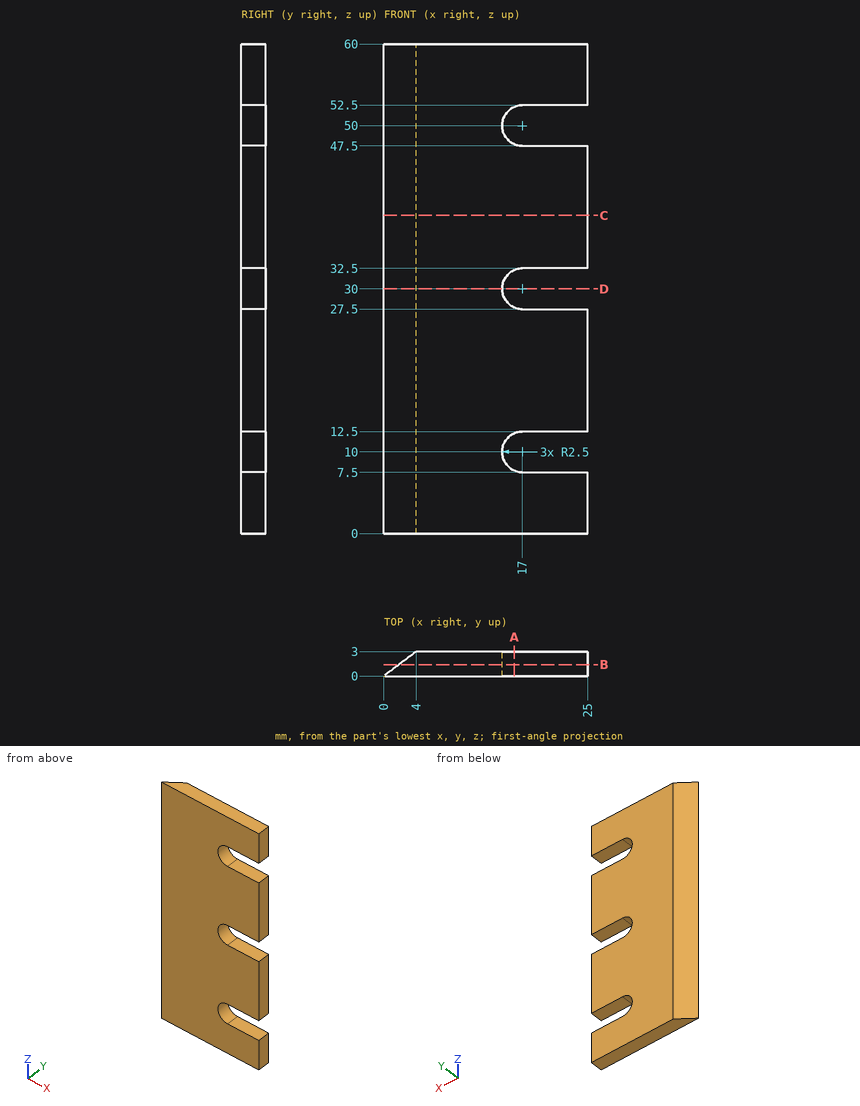
Could you check a few things on this drawing? It's one solid part, dimensions in mm from its lowest x, y, z. Give positions to 0.01 mm unless a question says otherwise; leave off trailing zeros. Write each loop counter-clockwise with the first axis right and the second up, starting at its lowest first coordinate (ties: lowest second). Pieces come first, ordered by that corner, then holes. Notation, with made-up numbers: M 22,41 L 78,41 A14 ccw 78,62 Z; hole C 4.5,80 d9. An arc over 180 degrees is marked long. Put each result on its own line as item: value. Start each with the question number.
Item 1: Will this pin go through, and if not, where does the flat tip stop? pin 1 (1 mm diameter, centred on x = 20, y = 2.5, fed in from -Z).
Item 2: If we section it at B-B, the plane y = 1.4: Write out the boundary of the cut face in (x, z), then the cut area to 3 significant figures.
Item 3: If we section it at A-A, the plane x = 16: Write out the boundary of the cut face in (y, z).
Item 4: If we section it at C-C, the plane z = 39: Write out the boundary of the cut face in (x, y), then the cut area to 3 significant figures.
Item 5: I need wall thicknesses on L1, parallel to Z at x = 18.75, y = 2.75; L2, parallel to X at y = 1.4, z = 42.5; L3, parallel to X at y = 2.1, z = 6. Which ranges of each line are inside material? Lowest first, please. Write a range as from..to.
Item 6: If we section it at D-D, the plane z = 30: Write out the boundary of the cut face in (x, y), then the cut area to 3 significant figures.
Values:
1. pin 1: z = 0
2. outline: M 1.87,0 L 25,0 L 25,7.5 L 17,7.5 A2.5 cw 17,12.5 L 25,12.5 L 25,27.5 L 17,27.5 A2.5 cw 17,32.5 L 25,32.5 L 25,47.5 L 17,47.5 A2.5 cw 17,52.5 L 25,52.5 L 25,60 L 1.87,60 Z
2. area: 1,240 mm²
3. outline: M 0,0 L 3,0 L 3,7.71 L 0,7.71 Z; M 0,12.29 L 3,12.29 L 3,27.71 L 0,27.71 Z; M 0,32.29 L 3,32.29 L 3,47.71 L 0,47.71 Z; M 0,52.29 L 3,52.29 L 3,60 L 0,60 Z
4. outline: M 0,0 L 25,0 L 25,3 L 4,3 Z
4. area: 69.0 mm²
5. L1: 0..7.5, 12.5..27.5, 32.5..47.5, 52.5..60
5. L2: 1.87..25
5. L3: 2.8..25
6. outline: M 0,0 L 14.5,0 L 14.5,3 L 4,3 Z
6. area: 37.5 mm²
